Source: CAD feature listing. Evaluate the final solid. Frame: model axes, mm. Face numbers are marked on the shaded views. A direction names the side the tool comes from. Coordinates: 2 decimals unless noted, no trailing zeros. Order: outer loops, then holes, each group sorted by start corner. A loop starts at its lowest first (then second) coordinate and runs counter-clockwise, first axis right, second up.
Item 1: Section C-C on y = -24. Return the cut outline in (x, z), then the cut area to 3 significant figures.
Item 2: Reachability of the marked faces 4, 5 and 6 from +Z, -Z, +X, -X, +Y, -Y: full face, straight path, thin tool, end or side. Return the list, or none.
Item 3: Section A-A on z = 19.5. Return the cut outline in (x, y), then the cut area to 3 significant figures.
Item 4: Section B-B on x = -31. Return the cut outline in (y, z).
Item 5: Mould query, pull axis Z, two halves, no side actions, for the marked faces 1, 2 and 3. Classes: released by +Z, released by -Z, zero draft, split by the parting line, or undercut.
Item 6: Contact query for flat-ended pins moving along their axis: P1, Ø10, axis at x = -57.5, z = 20.5, coming from the +Y side; P2, Ø3, axis at y = -27.5, z = 0.5, coming from the -X side; P3, Ø4, axis at x = -60, y = -30, coming from the -Z side; P4, Ø6.5, axis at x = -57, y = -28.5, coming from the +Z side. Output: stop coordinate, or through.
Item 7: Ray query, line 1 (X direction, y = -14, z = 35); line 2 (X direction, y = -42.5, z = 22.5); line 3 (Z direction, x = -12, y = -45). Return the intervals inside material, ascending.
Item 8: Section D-D on y = -32. Return the cut outline in (x, z), then the cut area to 3 significant figures.
from build123d import *

# Parameters (mm, degrees)
F0_W     = 53.24851
F0_H     = 51.189933
F1_DEPTH = 50.8
F2_R     = 7.591655
F3_DEPTH = 50.8
F4_W     = 19.213377
F4_H     = 18.938902
F5_DEPTH = 12.7
F6_R     = 14.591229
F7_DEPTH = 12.7


with BuildPart() as f1:
    # F0 (on Front) → F1 (new body)
    with BuildSketch(Plane.XZ):
        with Locations((-26.624255, 25.594966)):
            Rectangle(F0_W, F0_H)
    extrude(amount=F1_DEPTH)

    # F2 (on face) → F3 (cut)
    with BuildSketch(Plane.XZ.offset(50.8)):
        with Locations((-27.173208, 25.114631)):
            Circle(F2_R)
    extrude(amount=-F3_DEPTH, mode=Mode.SUBTRACT)

    # F4 (on face) → F5 (join)
    with BuildSketch(Plane(origin=(-53.24851, 0, 0), x_dir=(0, -1, 0), z_dir=(-1, 0, 0))):
        with Locations((25.800821, 24.702916)):
            Rectangle(F4_W, F4_H)
    extrude(amount=F5_DEPTH)

    # F6 (on face) → F7 (join)
    with BuildSketch(Plane(origin=(0, 0, 0), x_dir=(1, 0, 0), z_dir=(0, 0, -1))):
        with Locations((-26.487015, 24.977392)):
            Circle(F6_R)
    extrude(amount=F7_DEPTH)


solid = f1.part
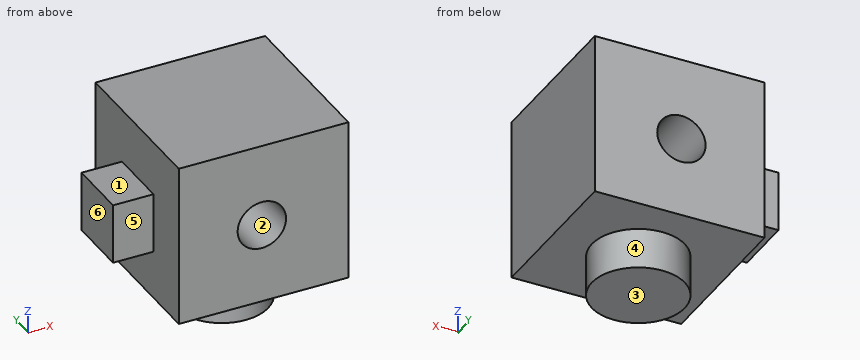
Answer list:
1. outline: (-65.95, 15.23) - (-53.25, 15.23) - (-53.25, 0) - (-41.05, 0) - (-41.05, -12.7) - (-11.93, -12.7) - (-11.93, 0) - (0, 0) - (0, 51.19) - (-53.25, 51.19) - (-53.25, 34.17) - (-65.95, 34.17) - close; hole circle Ø15.18 at (-27.17, 25.11)
1. area: 3,160 mm2
2. face 4: -Z
2. face 5: +Z, -Z, -X, -Y
2. face 6: +Z, -Z, -X, +Y, -Y
3. outline: (-65.95, -35.41) - (-53.25, -35.41) - (-53.25, -50.8) - (-32.28, -50.8) - (-32.28, 0) - (-53.25, 0) - (-53.25, -16.19) - (-65.95, -16.19) - close; (-22.06, -50.8) - (0, -50.8) - (0, 0) - (-22.06, 0) - close
3. area: 2,430 mm2
4. outline: (-50.8, 0) - (-38.85, 0) - (-38.85, -12.7) - (-11.1, -12.7) - (-11.1, 0) - (0, 0) - (0, 18.56) - (-50.8, 18.56) - close; (-50.8, 31.67) - (0, 31.67) - (0, 51.19) - (-50.8, 51.19) - close
5. face 1: released by +Z
5. face 2: undercut
5. face 3: released by -Z
6. P1: stops at y = 0
6. P2: stops at x = -53.25
6. P3: stops at z = 15.23
6. P4: stops at z = 34.17
7. line 1: x = -53.25 to 0
7. line 2: x = -53.25 to -34.3, -20.05 to 0
7. line 3: z = 0 to 51.19
8. outline: (-65.95, 15.23) - (-53.25, 15.23) - (-53.25, 0) - (-39.28, 0) - (-39.28, -12.7) - (-13.7, -12.7) - (-13.7, 0) - (0, 0) - (0, 51.19) - (-53.25, 51.19) - (-53.25, 34.17) - (-65.95, 34.17) - close; hole circle Ø15.18 at (-27.17, 25.11)
8. area: 3,110 mm2
